Verification items for the finished model (mm, model axes). A direction names the side the tool comes from. Give positions to 0.01 mm unless a question says otherwise; leave off trailing zeros. Loops run counter-clockwise (first coordinate to the right, second up) from the corner with the lowest first, then second, coordinate; pieces in that order, holes last. Notation, with made-up numbers: (59, 75.5) - (102, 75.5) arc R35 ccw to (102, 113.5) - close; hole circle Ø5 at (14.25, -30.75). An arc over 180 degrees is marked (long way). One line per item, written item: value. Start each with the question number.
1. Access from +Z, -Z, +X, -X, +Y, -Y to the whole of each face (thin tool, end or side, straight path). Record for faces 4 (the flat face through (10, 1, -15)), 5 (the cylindrical face through (0.301, 1.521, -19.715)).
2. Sectioned sample at C-C (x = 5). Record the cut outline in (y, z), plus the area to 3 significant figures.
3. Sectioned sample at D-D (y = 1.8). Record the cut outline in (x, z), plus the area to 3 significant figures.
4. Gauge pin test, flat ends, axial feed: pin 1 (8 mm diameter, centred on x = 4, z = -4, fed in from +Y); pin 2 (0.9 mm diameter, centred on x = 13.5, y = 1.5, fed in from -Z). Record the tip position at first contact, or that the pin passes through.
5. Sectioned sample at B-B (x = 15). Record the cut outline in (y, z), plus the area to 3 significant figures.
6. Sectioned sample at A-A (z = -15). Record the cut outline in (x, y).
7. Mould release check, pull along Z, two halves, no side actions. Record for faces 1 (the cylindrical face through (5.07, 1.48, -16.5)), 2 (the flat face through (10, 1, 0)), 3 (the flat face through (15, 1, -10)): pulls with the +Z half, pulls with the -Z half, needs draft (parallel to the pull), parting line crosses it, or undercut.
8. Scan lines: L1, parallel to X at y = 1.05, z = -5; L2, parallel to Z at x = 6, y = 1.75; L3, parallel to X at y = 0.4, z = -4.5. Record each from-to range of solid material in increasing order. Write a range as [from, to].
from build123d import *

# Parameters (mm, degrees)
SKETCH1_R           = 1.5
BOSS_EXTRUDE1_DEPTH = 3
FILLET1_R           = 1
FILLET2_R           = 1


with BuildPart() as part:
    # Sketch1 → Boss-Extrude1 (new body)
    with BuildSketch(Plane(origin=(0, 0, 0), x_dir=(1, 0, 0), z_dir=(0, 1, 0))):
        Polygon((0, 0), (10, 0), (20, 0), (20, 10), (10, 10), (10, 20), (0, 20), align=None)
        with Locations(Location((5, 15, 0), (0, 0, 270))):
            Circle(SKETCH1_R, mode=Mode.SUBTRACT)
        with Locations(Location((5, 5, 0), (0, 0, 270))):
            Circle(SKETCH1_R, mode=Mode.SUBTRACT)
        with Locations(Location((15, 5, 0), (0, 0, 270))):
            Circle(SKETCH1_R, mode=Mode.SUBTRACT)
    extrude(amount=BOSS_EXTRUDE1_DEPTH)

    # Fillet1
    fillet1_edges = [part.edges().sort_by_distance(p)[0] for p in [
        (10, 1.5, -10),
    ]]
    fillet(fillet1_edges, radius=FILLET1_R)

    # Fillet2
    fillet2_edges = [part.edges().sort_by_distance(p)[0] for p in [
        (0, 1.5, -20),
        (10, 1.5, -20),
        (20, 1.5, -10),
        (20, 1.5, 0),
        (0, 1.5, 0),
    ]]
    fillet(fillet2_edges, radius=FILLET2_R)


solid = part.part
Results are:
1. face 4: -Z, +X, +Y, -Y
1. face 5: -Z, -X, +Y, -Y
2. outline: (0, -20) - (3, -20) - (3, -16.5) - (0, -16.5) - close; (0, -13.5) - (3, -13.5) - (3, -6.5) - (0, -6.5) - close; (0, -3.5) - (3, -3.5) - (3, 0) - (0, 0) - close
2. area: 42.0 mm^2
3. outline: (0, -19) arc R1 ccw to (1, -20) - (9, -20) arc R1 ccw to (10, -19) - (10, -11) arc R1 cw to (11, -10) - (19, -10) arc R1 ccw to (20, -9) - (20, -1) arc R1 ccw to (19, 0) - (1, 0) arc R1 ccw to (0, -1) - close; hole circle Ø3 at (5, -15); hole circle Ø3 at (5, -5); hole circle Ø3 at (15, -5)
3. area: 278 mm^2
4. pin 1: stops at y = 3
4. pin 2: stops at z = -10
5. outline: (0, -10) - (3, -10) - (3, -6.5) - (0, -6.5) - close; (0, -3.5) - (3, -3.5) - (3, 0) - (0, 0) - close
5. area: 21.0 mm^2
6. outline: (0, 0) - (3.5, 0) - (3.5, 3) - (0, 3) - close; (6.5, 0) - (10, 0) - (10, 3) - (6.5, 3) - close
7. face 1: undercut
7. face 2: pulls with the +Z half
7. face 3: pulls with the -Z half
8. L1: x = [0, 3.5], [6.5, 13.5], [16.5, 20]
8. L2: z = [-20, -16.12], [-13.88, -6.12], [-3.88, 0]
8. L3: x = [0, 3.59], [6.41, 13.59], [16.41, 20]
